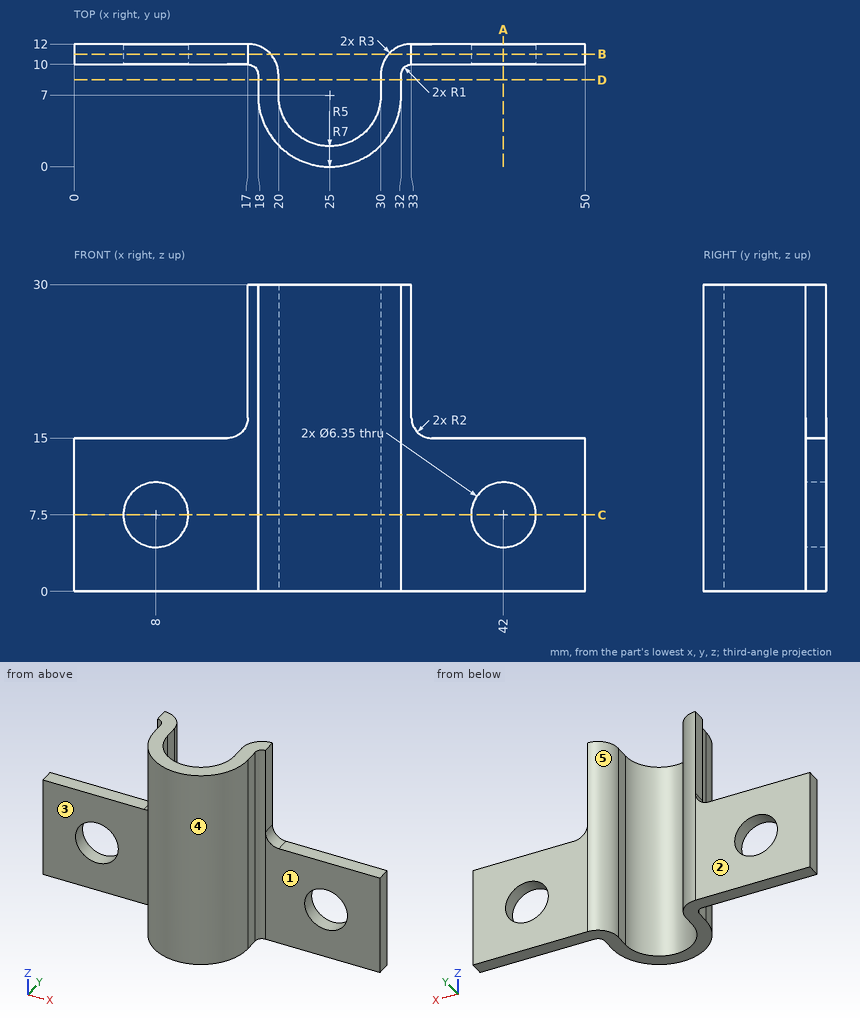
Design review of the part shown in the three views and the two pictorial views. Dimensions are in mm from the part's minimum x, y and z. A direction names the side the tool comes from. Coordinates: 2 decimals unless noted, no trailing zeros. Order: outer loops, then holes, each group sorted by start corner. A loop starts at its lowest first (then second) coordinate and runs counter-clockwise, first axis right, second up. Notation, with made-up numbers: (-6.5, 10) -> (36.5, 10) arc R19 cw to (36.5, 36) -> close; hole circle Ø10 at (36.25, -21). An arc over 180 degrees is marked (long way). Use one line per item in the form item = value. Start each with the question number.
(1) Add section A-A on x = 42. State the section outline as (y, z) points (3 decimals), plus the area to 3 significant figures.
(2) Add section D-D on y = 8.5. State the section outline as (x, z) points, plus the area to 3 significant figures.
(3) The part is to be moulded in two halves that separate along X. For the marked faces 3, 4 and 5, say which applies: +X half, -X half, draft (parallel to the pull), parting line (faces both ways), or undercut.
(4) Add section B-B on y = 11. State the section outline as (x, z) points (3 decimals).
(5) Add section C-C on z = 7.5. State the section outline as (x, y) points (3 decimals), plus the area to 3 significant figures.
(6) For probe 1 along Z at (x, y) = (42, 11.65) (3 decimals); probe 2 along Y at (x, z) = (39, 4.5); probe 3 along X at (y, z) = (4.5, 27.75), list the stretches that pass through material, from the lowest coordinate up.
(7) For the marked faces 1 and 2, list the 3-axis set-ups (+Z, -Z, +X, -X, +Y, -Y) from which the entire face can be reached by the end or side of a thin tool; tool diameter is ignored.
(8) Insertion check: pin 1 (1.6 mm diameter, centred on y = 8, z = 21, fed in from -X); pin 2 (1.6 mm diameter, centred on y = 8, z = 16, fed in from +X); pin 3 (4 mm diameter, centred on y = 4, z = 3.5, fed in from -X); pin 4 (1.5 mm diameter, centred on x = 12.5, y = 10.5, fed in from -Z). Each pin has a flat end and moves straight along its axis. Give the tip position at first contact, or say it passes through.
Answer block:
q1.outline = (10, 0) -> (12, 0) -> (12, 4.325) -> (10, 4.325) -> close; (10, 10.675) -> (12, 10.675) -> (12, 15) -> (10, 15) -> close
q1.area = 17.3 mm²
q2.outline = (18, 0) -> (20, 0) -> (20, 30) -> (18, 30) -> close; (30, 0) -> (32, 0) -> (32, 30) -> (30, 30) -> close
q2.area = 120 mm²
q3.face_3 = draft
q3.face_4 = parting line
q3.face_5 = undercut
q4.outline = (0, 0) -> (19.236, 0) -> (19.236, 30) -> (17, 30) -> (17, 17) arc R2 cw to (15, 15) -> (0, 15) -> close; (30.764, 0) -> (50, 0) -> (50, 15) -> (35, 15) arc R2 cw to (33, 17) -> (33, 30) -> (30.764, 30) -> close; hole circle Ø6.35 at (8, 7.5); hole circle Ø6.35 at (42, 7.5)
q5.outline = (0, 10) -> (4.825, 10) -> (4.825, 12) -> (0, 12) -> close; (11.175, 10) -> (17, 10) arc R1 cw to (18, 9) -> (18, 7) arc R7 ccw to (32, 7) -> (32, 9) arc R1 cw to (33, 10) -> (38.825, 10) -> (38.825, 12) -> (33, 12) arc R3 ccw to (30, 9) -> (30, 7) arc R5 cw to (20, 7) -> (20, 9) arc R3 ccw to (17, 12) -> (11.175, 12) -> close; (45.175, 10) -> (50, 10) -> (50, 12) -> (45.175, 12) -> close
q5.area = 101 mm²
q6.probe_1 = 0 to 4.325, 10.675 to 15
q6.probe_2 = 10 to 12
q6.probe_3 = 18.46 to 20.67, 29.33 to 31.54
q7.face_1 = +Z, -Z, +X, -Y
q7.face_2 = +Z, -Z, +X, -X, +Y
q8.pin_1 = 18
q8.pin_2 = 32
q8.pin_3 = 18.07
q8.pin_4 = 0
